Design review of the part built by this model. Coordinates are the model's own, in mm. Give positions to 0.01 mm unless a question says otherwise; leave off trailing zeros. Write each loop counter-clockwise with the first axis right and the second up, starting at its lowest first coordinate (ties: lowest second). Pieces come first, ordered by that corner, then holes. Notation, with made-up numbers: (88, 26.5) - (138, 26.5) arc R22 ccw to (138, 48.5) - close; hole circle Ø6 at (-28, 18). An arc over 180 degrees is marked (long way). Use a Markdown table: item, result. Add a question column.
Autodesk Inventor part; units mm, degrees
ref_plane "YZ Plane" through (0, 0, 0) normal (1, 0, 0) x (0, 1, 0)
ref_plane "XZ Plane" through (0, 0, 0) normal (0, 1, 0) x (-1, 0, 0)
ref_plane "XY Plane" through (0, 0, 0) normal (0, 0, 1) x (1, 0, 0)
sketch "スケッチ1" plane through (0, 0, 0) normal (0, 1, 0) x (-1, 0, 0)
  line L0 (4.95, 23.5) -> (-8.05, 23.5)
  line L1 (-8.05, 23.5) -> (-8.05, -23.5)
  line L2 (-8.05, -23.5) -> (4.95, -23.5)
  line L3 (4.95, -23.5) -> (4.95, 23.5)
  point P0 (0, 0)
  dimension "d12" = 4.95
  dimension "d13" = 8.05
  dimension "d14" = 47
  dimension "d15" = 23.5
extrude "押し出し1" add sketch "スケッチ1" against normal blind 1
sketch "スケッチ2" plane through (0, 0, 0) normal (0, 1, 0) x (1, 0, 0)
  circle A0 centre (-2.95, 21.5) radius 1
  line L0 (8.05, -23.5) -> (8.05, 23.5)
  line L1 (8.05, 23.5) -> (-4.95, 23.5)
  circle A1 centre (-2.95, -21.5) radius 1
  line L2 (-4.95, -23.5) -> (8.05, -23.5)
  point P0 (0, 0)
  dimension "d4" = 2
  dimension "d5" = 11
  dimension "d6" = 2
  dimension "d7" = 2
  dimension "d8" = 11
  dimension "d9" = 2
extrude "押し出し2" cut sketch "スケッチ2" against normal blind 1
equation "\"d7\" = d4"
equation "\"d8\" = d5"
equation "\"d9\" = d6"
properties part number "kiban"
(1) For line 1 along Z through (x, y) = (-2.95, -0.35); line 2 along X through (y, z) = (-0.3, 21.5); line 3 along Z through (x, y) = (-2.5, -0.8), list the stretches that pass through material, from the lowest coordinate up.
(2) Add section B-B (z = 21.5). State the section outline as (x, y) points, and give its area (3 significant figures).
(3) Add section A-A (x = -2.95). State the section outline as (y, z) points, and give its area (3 significant figures).
(4) Mouldability with a two-part tool opening along Z and no side actions: class faces 1 (the face through (-2.49, -0.49, 22.39)), 2 (the face through (8.05, -0.5, 0.3)), 3 (the face through (-2.49, -0.49, -20.61)), 4 (the face through (1.5, -0.5, 23.5)) as +Z half, -Z half, draft (parallel to the pull), parting line (faces both ways), or undercut.
Answers follow:
| question | item | result |
|---|---|---|
| 1 | line 1 | -23.5 to -22.5, -20.5 to 20.5, 22.5 to 23.5 |
| 1 | line 2 | -4.95 to -3.95, -1.95 to 8.05 |
| 1 | line 3 | -23.5 to -22.39, -20.61 to 20.61, 22.39 to 23.5 |
| 2 | outline | (-4.95, -1) - (-3.95, -1) - (-3.95, 0) - (-4.95, 0) - close; (-1.95, -1) - (8.05, -1) - (8.05, 0) - (-1.95, 0) - close |
| 2 | area | 11.0 mm^2 |
| 3 | outline | (-1, -23.5) - (0, -23.5) - (0, -22.5) - (-1, -22.5) - close; (-1, -20.5) - (0, -20.5) - (0, 20.5) - (-1, 20.5) - close; (-1, 22.5) - (0, 22.5) - (0, 23.5) - (-1, 23.5) - close |
| 3 | area | 43.0 mm^2 |
| 4 | face 1 | undercut |
| 4 | face 2 | draft |
| 4 | face 3 | undercut |
| 4 | face 4 | +Z half |
